Geometry check sheet. Reference: drawing and pictorial views, mm from the part's lowest x, y, z. A direction names the side the tool comes from. Coordinates: 2 decimals unless noted, no trailing zeros. Loops run counter-clockwise (first coordinate to the right, second up) from the corner with the lowest first, then second, coordinate; pieces in that order, holes last. Notation, with made-up numbers: (-0.5, -26.75) -> (15.5, -26.75) arc R24 cw to (15.5, -7.75) -> close; hole circle Ø2 at (-17, -24). An arc over 180 degrees is marked (long way). Use CSV: the item, a comma, the result in double quotes.
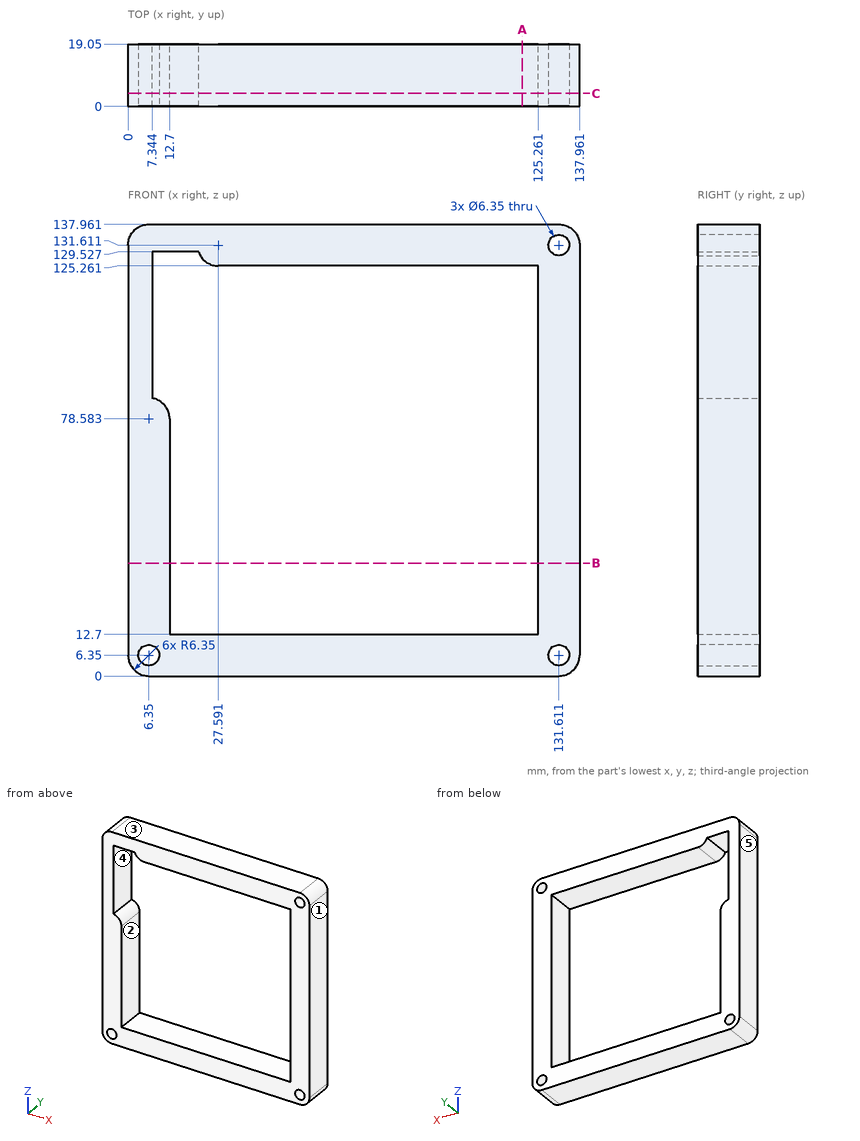
1) Cross-section at C-C on y = 4. Give the number of separate pieces and of enclosed holes in the cut face, and give its area (3 significant figures).
Answer below:
separate pieces,"1"
enclosed holes,"4"
area,"5,940 mm²"
2) Access from +Z, -Z, +X, -X, +Y, -Y to the whole of each face (thin tool, end or side, straight path). Record for the marked faces 4 and 5.
Answer below:
face 4,"+Y, -Y"
face 5,"+Z, -Z, -X, +Y, -Y"
3) Draft check along X on the marked faces 1, 2 and 3. Enter one of: released by +X, released by -X, zero draft, split by the parting line, or undercut.
Answer below:
face 1,"released by +X"
face 2,"undercut"
face 3,"zero draft"
4) Thickness scan on line 1 along X through (y, z) = (8.5, 6.35) (1 decimal); line 2 along X through (y, z) = (4, 69). Record the ranges inside material, lowest first. Write a range as from..to.
Answer below:
line 1,"x = 0..3.2, 9.5..128.4, 134.8..138"
line 2,"x = 0..12.7, 125.26..137.96"
5) Cross-section at B-B on z = 34.5. Record the boundary of the cut face in (x, y), and give its area (3 significant figures).
Answer below:
outline,"(0, 0) -> (12.7, 0) -> (12.7, 19.05) -> (0, 19.05) -> close; (125.26, 0) -> (137.96, 0) -> (137.96, 19.05) -> (125.26, 19.05) -> close"
area,"484 mm²"
6) Cross-section at A-A on x = 120.5. Record the boundary of the cut face in (y, z).
Answer below:
outline,"(0, 0) -> (19.05, 0) -> (19.05, 12.7) -> (0, 12.7) -> close; (0, 125.26) -> (19.05, 125.26) -> (19.05, 137.96) -> (0, 137.96) -> close"
